```python
from build123d import *

# Parameters (mm, degrees)
SKETCH1_W                  = 6.35
SKETCH1_H                  = 12.7
BOSS_EXTRUDE1_DEPTH        = 240.03
CUT_EXTRUDE_THIN1_DEPTH    = 241.449606779
F_35_0_11_DIAMETER_HOLE1_D = 2.794
F_6_CLEARANCE_HOLE1_D      = 3.6576


with BuildPart() as part:
    # Sketch1 → Boss-Extrude1 (new body)
    with BuildSketch(Plane(origin=(0, 0, 0), x_dir=(1, 0, 0), z_dir=(0, 1, 0))):
        with Locations((3.175, 6.35)):
            Rectangle(SKETCH1_W, SKETCH1_H)
    extrude(amount=BOSS_EXTRUDE1_DEPTH)

    # Sketch2 → Cut-Extrude-Thin1 (cut, through all)
    with BuildSketch(Plane.ZY):
        Polygon((0, 233.68), (-9.525, 233.68), (-9.525, 240.03), (-9.52510033, 240.03), (-9.52510033, 233.67989967), (0, 233.67989967), align=None)
        Polygon((0, 143.51), (-6.35, 143.51), (-6.35, 233.68), (-6.35010033, 233.68), (-6.35010033, 143.50989967), (0, 143.50989967), align=None)
        Polygon((0, 137.16), (-6.35, 137.16), (-6.35, 74.93), (0, 74.93), (0, 74.93010033), (-6.34989967, 74.93010033), (-6.34989967, 137.15989967), (0, 137.15989967), align=None)
        Polygon((0, 68.58), (-6.35, 68.58), (-6.35, 6.35), (0, 6.35), (0, 6.35010033), (-6.34989967, 6.35010033), (-6.34989967, 68.57989967), (0, 68.57989967), align=None)
    extrude(amount=-CUT_EXTRUDE_THIN1_DEPTH, mode=Mode.SUBTRACT)


with BuildPart() as cut_extrude_thin1_kept_piece:
    # of the separate pieces the step leaves, the one the design keeps (cut_extrude_thin1_pieces_kept)
    add(part.part.solids().sort_by_distance((0, 0, 0))[0])

    # #35 (0.11) Diameter Hole1 (through all)
    with Locations(Plane.XY):
        with Locations((3.175, 140.335), (3.175, 71.755), (3.175, 3.174949835)):
            Hole(F_35_0_11_DIAMETER_HOLE1_D / 2)

    # #6 Clearance Hole1 (through all)
    with Locations(Plane.XY.offset(-9.52510033)):
        with Locations((3.175, 236.854949835)):
            Hole(F_6_CLEARANCE_HOLE1_D / 2)


solid = cut_extrude_thin1_kept_piece.part
```
Build history of the part. All positions in model axes, mm. A direction names the side the tool comes from. Round coordinates to 2 decimals unless told otherwise and drop trailing zeros. Write each loop counter-clockwise with the first axis right and the second up, starting at its lowest first coordinate (ties: lowest second). Pieces come first, ordered by that corner, then holes.
1) Mould opens along Y. For faces 1 (the cylindrical face through (4.523, 238.091, -11.135)), 2 (the flat face through (3, 0, -6)), 3 (the flat face through (3, 118, -12.7)) say: +Y half, -Y half, draft (parallel to the pull), parting line (faces both ways), or undercut.
2) 3-axis set-ups, long thin cutter, end or side, ignore diameter. For faces 4 (the flat face through (3, 143.51, -3)), 5 (the flat face through (3, 106, -6.35)), 6 (the flat face through (0, 118, -10)): which of +Z, -Z, +X, -X, +Y, -Y reach the whole face in a straight line?
3) Pin check, flat tips, straight feed: pin 1 (3 mm diameter, centred on x = 3, z = -2.5, fed in from +Y); pin 2 (1 mm diameter, centred on x = 4, z = -8, fed in from +Y); pin 3 (3 mm diameter, centred on x = 4, y = 128, fed in from +Z). Stop position of each tip, or through.
4) Drill centre lines: probe 1 along Y at (x, z) = (3.5, -3.75); probe 2 along Y at (x, z) = (3.5, -11); probe 3 along Y at (x, z) = (0.5, -5.25). Where is each one in solid material? Low to high.
5) Band-saw the part on B-B, the plane y = 47. List the corners of the cut face in (x, z).
6) Band-saw the part on A-A, the plane z = -3. List the corners of the cut face in (x, y) (3 decimals).
Ans:
1. face 1: undercut
1. face 2: -Y half
1. face 3: draft
2. face 4: +Z, +X, -X, +Y
2. face 5: +Z, +X, -X
2. face 6: +Z, -Z, -X, +Y, -Y
3. pin 1: stops at y = 143.51
3. pin 2: stops at y = 233.68
3. pin 3: stops at z = -6.35
4. probe 1: y = 0 to 1.82, 4.53 to 6.35, 68.58 to 70.4, 73.11 to 74.93, 137.16 to 138.98, 141.69 to 143.51
4. probe 2: y = 0 to 1.82, 4.53 to 70.4, 73.11 to 138.98, 141.69 to 235.06, 238.65 to 240.03
4. probe 3: y = 0 to 6.35, 68.58 to 74.93, 137.16 to 143.51
5. outline: (0, -12.7) - (6.35, -12.7) - (6.35, -6.35) - (0, -6.35) - close
6. outline: (0, 0) - (6.35, 0) - (6.35, 6.35) - (0, 6.35) - close; (0, 68.58) - (6.35, 68.58) - (6.35, 74.93) - (0, 74.93) - close; (0, 137.16) - (6.35, 137.16) - (6.35, 143.51) - (0, 143.51) - close; hole circle Ø2.794 at (3.175, 3.175); hole circle Ø2.794 at (3.175, 71.755); hole circle Ø2.794 at (3.175, 140.335)
